Could you check a few things on this drawing? It's one solid part, dimensions in mm from its lowest x, y, z. Round coordinates to 2 decimals unless told otherwise and drop trailing zeros. Write each loop counter-clockwise with the first axis right and the second up, starting at its lowest first coordinate (ties: lowest second). Pieces come first, ordered by that corner, then holes. Notation, with made-up numbers: (41.5, 72) - (81.5, 72) arc R23 ccw to (81.5, 91) - close; hole circle Ø5 at (-21, 26.5). An arc over 180 degrees is marked (long way). Use one line per item in the form item = value. Start each with the question number.
1. I want a section at B-B, the plane z = 35. List the corners of the cut face in (x, y) for me.
2. I want a section at A-A, the plane x = 35. List the corners of the cut face in (y, z) for me, plus the area to 3 significant figures.
3. Will these pins go through, and if not, where does the flat tip stop? pin 1 (1.5 mm diameter, centred on y = 1.5, z = 60, fed in from +X); pin 2 (13.5 mm diameter, centred on x = 35, z = 35, fed in from -Y); pin 3 (1.5 mm diameter, centred on x = 9.5, y = 2, fed in from -Z); pin 4 (2.5 mm diameter, centred on y = 2, z = 17.5, fed in from -X).
4. I want a section at D-D, the plane x = 51.5. List the corners of the cut face in (y, z) for me (1 decimal).
5. I want a section at C-C, the plane z = 62.5. List the corners of the cut face in (x, y) for me, plus the area to 3 significant figures.
6. If I drill on line 1 along Z through (x, y) = (51, 3.2) (1 decimal); line 2 along Z through (x, y) = (35, 1.7); line 3 along X through (y, z) = (0.5, 48) (1 decimal), over which ranges is the centre line in solid material (lowest first)?
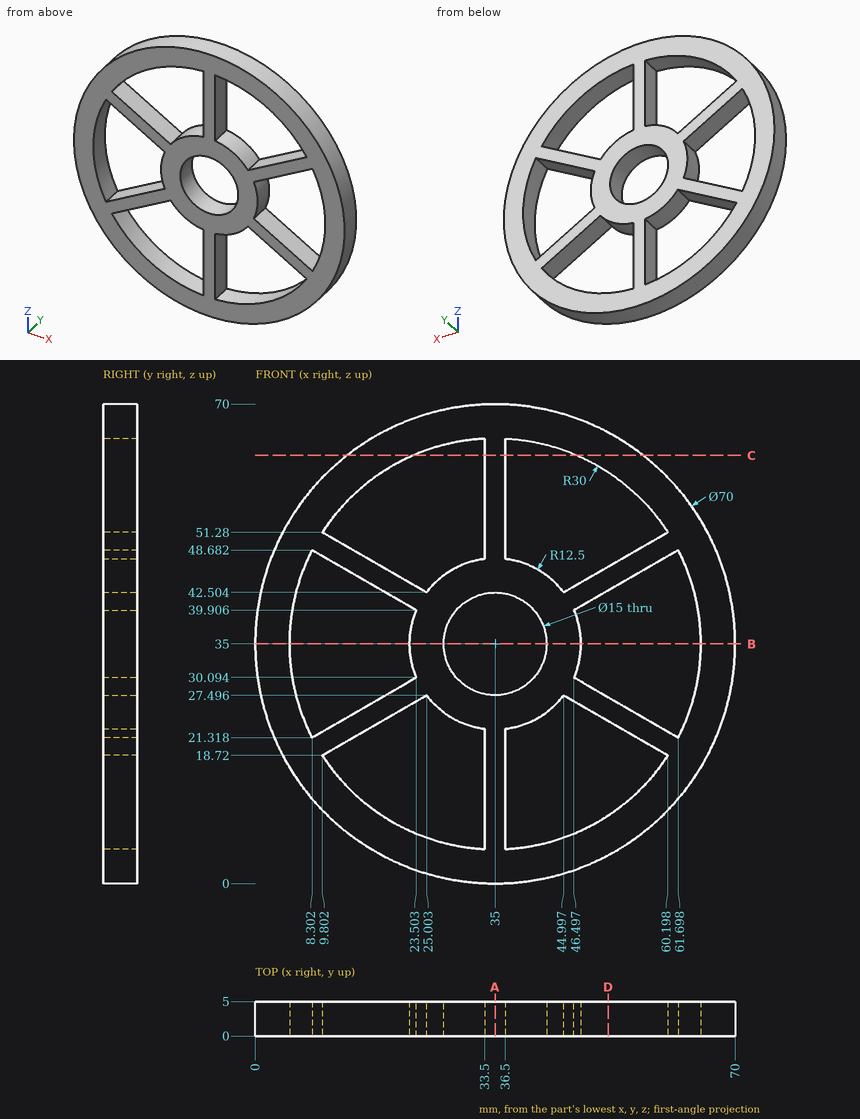
Model answer:
q1.outline = (0, 0) - (5, 0) - (5, 5) - (0, 5) - close; (22.5, 0) - (27.5, 0) - (27.5, 5) - (22.5, 5) - close; (42.5, 0) - (47.5, 0) - (47.5, 5) - (42.5, 5) - close; (65, 0) - (70, 0) - (70, 5) - (65, 5) - close
q2.outline = (0, 0) - (5, 0) - (5, 27.5) - (0, 27.5) - close; (0, 42.5) - (5, 42.5) - (5, 70) - (0, 70) - close
q2.area = 275 mm2
q3.pin_1 = 60.24
q3.pin_2 = through
q3.pin_3 = 10.25
q3.pin_4 = 4
q4.outline = (0, 4.1) - (5, 4.1) - (5, 9.9) - (0, 9.9) - close; (0, 23.7) - (5, 23.7) - (5, 27.2) - (0, 27.2) - close; (0, 42.8) - (5, 42.8) - (5, 46.3) - (0, 46.3) - close; (0, 60.1) - (5, 60.1) - (5, 65.9) - (0, 65.9) - close
q5.outline = (13.35, 0) - (23.01, 0) - (23.01, 5) - (13.35, 5) - close; (33.5, 0) - (36.5, 0) - (36.5, 5) - (33.5, 5) - close; (46.99, 0) - (56.65, 0) - (56.65, 5) - (46.99, 5) - close
q5.area = 112 mm2
q6.line_1 = 3.9 to 9.6, 24 to 27.5, 42.5 to 46, 60.4 to 66.1
q6.line_2 = 0 to 27.5, 42.5 to 70
q6.line_3 = 2.5 to 8, 9.5 to 15.5, 33.5 to 36.5, 54.5 to 60.5, 62 to 67.5
